Design review of the part built by this model. Coordinates are the model's own, in mm. A direction names the side the tool comes from. Round coordinates to 2 decimals unless told otherwise and drop trailing zeros. Loops run counter-clockwise (first coordinate to the right, second up) from the corner with the lowest first, then second, coordinate; pieces in that order, holes last. Notation, with made-up numbers: (6.25, 27) -> (42.25, 27) arc R15 cw to (42.25, 39) -> close; hole circle Ø2 at (-34.75, -23.75). An arc over 180 degrees is marked (long way). Answer as CSV lines item,"result". Start each with the question number.
(1) Machinability: for faces 1 (the face through (-15, 2, 2)), 2 (the face through (-11.115, 0.301, 4.521)), 3 (the face through (-0.57, 3.4, 1.52)), 4 (the face through (-11.099, 1.715, 4.521)), which of the approach directions +Z, -Z, +X, -X, +Y, -Y give a long, thin tool a straight path to every point of the face, cutting with its end or side? Answer none if there is none.
(2) To check wall thickness, follow line 1 (Y direction, x = -2, z = 2.1); line 2 (Z direction, x = -17, y = 1.85); line 3 (Y direction, x = -28, z = 0.75). State the ranges of each line that lie inside material, in increasing order. Write a range as from..to.
(3) For P1, Ø1.8, axis at x = -21.5, z = 3, coming from the +Y side; P2, Ø1, axis at x = -28.5, y = 2, coming from the -Z side; P3, Ø2, axis at x = -18.5, y = 1, coming from the +Z side, all flat-tipped, find the tip position at first contact; note any pin that passes through.
(4) Take a section at D-D, the plane x = -15.5. Write out the cut boundary in (y, z).
Autodesk Inventor part; units mm, degrees
ref_plane "YZ Plane" through (0, 0, 0) normal (1, 0, 0) x (0, 1, 0)
ref_plane "XZ Plane" through (0, 0, 0) normal (0, 1, 0) x (-1, 0, 0)
ref_plane "XY Plane" through (0, 0, 0) normal (0, 0, 1) x (1, 0, 0)
sketch "Sketch1" plane through (0, 0, 0) normal (0, 0, 1) x (1, 0, 0)
  line L0 (0, 0) -> (-4, 0)
  line L1 (-4, 0) -> (-4, 4)
  line L2 (-4, 4) -> (0, 4)
  line L3 (0, 4) -> (0, 0)
  line L4 (-4, 0) -> (-33, 0)
  line L5 (-33, 0) -> (-33, 2)
  line L6 (-33, 2) -> (-4, 2)
  line L7 (-4, 2) -> (-4, 0)
  dimension "d1" = 4
  dimension "d3" = 29
  dimension "d4" = 2
extrude "Soporte Hoja" add sketch "Sketch1" along normal blind 3
fillet "Cabeza" radius 2 3 edges at (0, 0, 1.5) (0, 4, 1.5) (-4, 4, 1.5)
fillet "Agarre Hoja" radius 1 2 edges at (-33, 0, 1.5) (-33, 2, 1.5)
sketch "Sketch2" plane through (0, 0, 3) normal (0, 0, 1) x (1, 0, 0)
  circle A0 centre (-2, 2) radius 0.5
  arc A1 (-2, 0) -> (-4, 2) centre (-2, 2) ccw
  point P0 (0, 0)
  dimension "d9" = 1
hole "Eje" at (-2, 2, 3) direction (0, 0, -1) diameter 1 end through all
sketch "Sketch3" plane through (0, 0, 3) normal (0, 0, 1) x (1, 0, 0)
  line L0 (-4, 2) -> (-32, 2)
  line L1 (-32, 0) -> (-2, 0)
  line L2 (-4, 2) -> (-32, 2)
  line L3 (-11.4, 2) -> (-11.4, 0)
  line L4 (-32, 0) -> (-2, 0)
  arc A0 (-2, 0) -> (-4, 2) centre (-2, 2) ccw
  circle A1 centre (-2, 2) radius 0.5
  point P0 (0, 0)
  dimension "d17" = 11.4
extrude "Soporte Deslizador" add sketch "Sketch3" along normal blind 3
fillet "Agarre Deslizador" radius 1 2 edges at (-11.4, 0, 4.5) (-11.4, 2, 4.5)
equation "\"d1\" = traba_cabeza_ancho"
equation "\"d3\" = traba_largo"
equation "\"d4\" = traba_hoja_ancho"
equation "\"d5\" = traba_hoja_grosor"
equation "\"d7\" = 0.5 * traba_cabeza_ancho"
equation "\"d8\" = 0.5 * traba_hoja_ancho"
equation "\"d10\" = traba_eje_diametro"
equation "\"d18\" = traba_deslizador_alto"
equation "\"d20\" = 0.5 * traba_hoja_ancho"
properties part number "Traba"
The answers:
1,face 1,"+Z, -Z, -X, +Y"
1,face 2,"+Z, -X, -Y"
1,face 3,"+Z, -Z, +X, +Y"
1,face 4,"+Z, -X, +Y"
2,line 1,"0..1.5, 2.5..4"
2,line 2,"0..3"
2,line 3,"0..2"
3,P1,"y = 2"
3,P2,"z = 0"
3,P3,"z = 3"
4,outline,"(0, 0) -> (2, 0) -> (2, 3) -> (0, 3) -> close"
